Verification items for this drawing (mm, ordinates from the low corner). A direction names the side the tool comes from. Round coordinates to 2 decimals unless told otherwise and drop trailing zeros. Order: outer loops, then holes, each group sorted by start corner. A loop starts at its lowest first (then second) coordinate and runs counter-clockwise, first axis right, second up. Notation, with made-up numbers: (-4, 27) - (36, 27) arc R15 cw to (36, 52) - close; hole circle Ø11 at (68.5, 18.25). An arc over 180 degrees is marked (long way). Return JSON: item names as keys, results as strings. Group by question number.
Q1. Sectioned sample at B-B, the plane z = 0.85. Record the cut outline in (x, y).
Q2. Material ranges on line 1 along Y through (x, z) = (7.7, 0.9); line 2 along Y through (x, z) = (7.7, 5.15); line 3 along Z through (x, y) = (4.25, 21.5), recorded low to high.
Q3. Sectioned sample at A-A, the plane x = 7.7. Record the cut outline in (y, z), then the cut area to 3 significant figures.
Q4. Draft check along Y on the marked faces 1, 2 and 3. Enter one of: pulls with the +Y half, pulls with the -Y half, needs draft (parallel to the pull), parting line crosses it, or undercut.
Q5. Gauge pin test, flat ends, axial feed: pin 1 Ø9 at (x, y) = (8, 15) entering from -Z; pin 2 Ø2 at (x, z) = (9.5, 2) entering from +Y; pin 3 Ø0.9 at (y, z) = (11, 5) entering from +X; pin 4 Ø8 at (x, y) = (7.7, 15.2) entering from -Z. Record the tip position at first contact, or that the pin passes through.
Q6. Tool access check on the marked faces 4, 5, 6 and 7. Record the directions out of +Z, -Z, +X, -X, +Y, -Y that give a thin tool (end or side, any length) a straight path to the whole face; none if there is none.
Q7. Sectioned sample at C-C, the plane y = 17.25. Record the cut outline in (x, z), then the cut area to 3 significant figures.
Q8. Sectioned sample at D-D, the plane y = 8.75. Record the cut outline in (x, z), then the cut area to 3 significant figures.
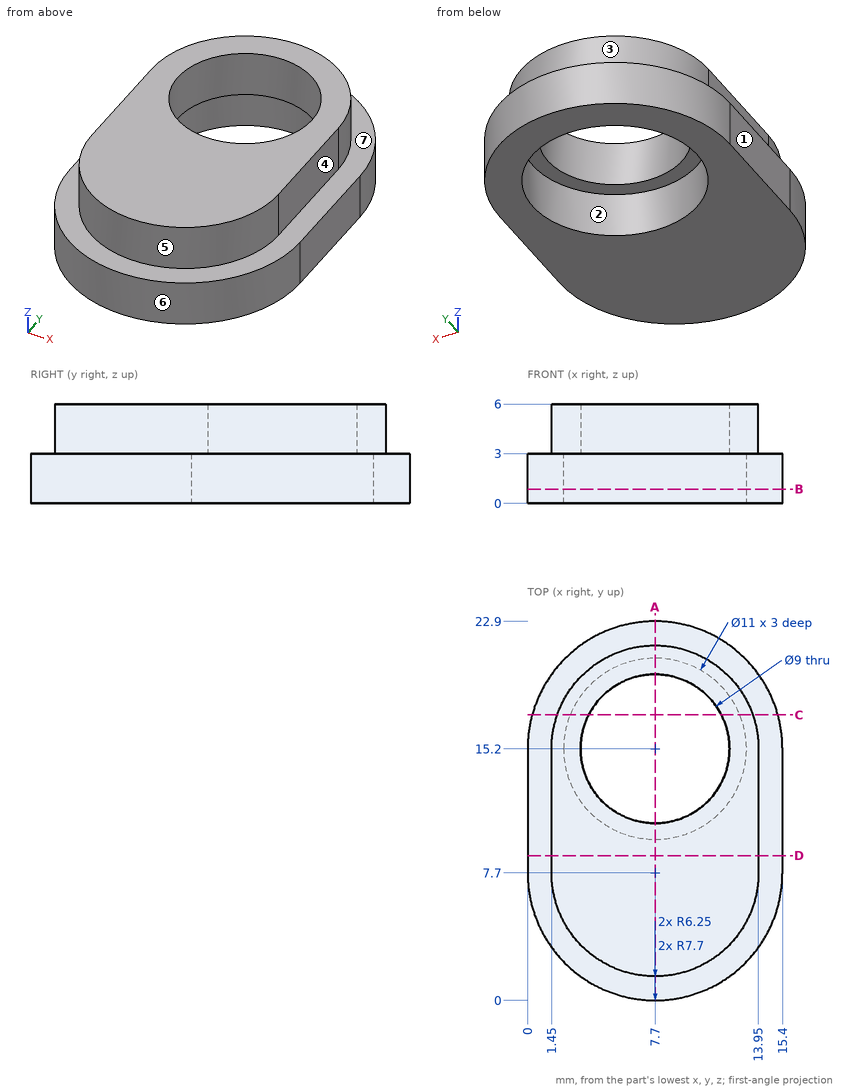
Reply:
{
 "1": {"outline": "(0, 7.7) arc R7.7 ccw to (15.4, 7.7) - (15.4, 15.2) arc R7.7 ccw to (0, 15.2) - close; hole circle Ø11 at (7.7, 15.2)"},
 "2": {"line 1": "0 to 9.7, 20.7 to 22.9", "line 2": "1.45 to 10.7, 19.7 to 21.45", "line 3": "0 to 3"},
 "3": {"outline": "(0, 0) - (9.7, 0) - (9.7, 3) - (10.7, 3) - (10.7, 6) - (1.45, 6) - (1.45, 3) - (0, 3) - close; (19.7, 3) - (20.7, 3) - (20.7, 0) - (22.9, 0) - (22.9, 3) - (21.45, 3) - (21.45, 6) - (19.7, 6) - close", "area": "68.7 mm^2"},
 "4": {"face 1": "needs draft", "face 2": "undercut", "face 3": "pulls with the +Y half"},
 "5": {"pin 1": "z = 3", "pin 2": "y = 22.86", "pin 3": "x = 13.95", "pin 4": "through"},
 "6": {"face 4": "+Z, +X, +Y, -Y", "face 5": "+Z, -Y", "face 6": "+Z, -Z, -Y", "face 7": "+Z"},
 "7": {"outline": "(0.28, 0) - (2.6, 0) - (2.6, 3) - (3.69, 3) - (3.69, 6) - (1.8, 6) - (1.8, 3) - (0.28, 3) - close; (11.71, 3) - (12.8, 3) - (12.8, 0) - (15.12, 0) - (15.12, 3) - (13.6, 3) - (13.6, 6) - (11.71, 6) - close", "area": "25.3 mm^2"},
 "8": {"outline": "(0, 0) - (15.4, 0) - (15.4, 3) - (13.95, 3) - (13.95, 6) - (1.45, 6) - (1.45, 3) - (0, 3) - close", "area": "83.7 mm^2"}
}
